from build123d import *
from build123d import SkipClean  # not in build123d's __all__

# Parameters (mm, degrees)
F1_DEPTH = 2
F2_R     = 6.75
F2_R_2   = 4
F3_DEPTH = 0.7
F4_SIZE2 = 1.5
F4_SIZE  = 3


with BuildPart() as f1:
    # F0 (on Top) → F1 (new body)
    with BuildSketch(Plane.XY):
        with BuildLine():
            ThreePointArc((0, 8.25), (-8.25, 0), (0, -8.25))
            Line((0, -8.25), (0, -14))
            ThreePointArc((0, -14), (4.5374051759, -13.2443178107), (8.5849765979, -11.05885061))
            ThreePointArc((8.5849765979, -11.05885061), (17.2671345057, -6.3709601788), (27, -4.75))
            ThreePointArc((27, -4.75), (36.7328654943, -6.3709601788), (45.4150234021, -11.05885061))
            ThreePointArc((45.4150234021, -11.05885061), (49.4625948241, -13.2443178107), (54, -14))
            Line((54, -14), (54, -8.25))
            ThreePointArc((54, -8.25), (62.25, 0), (54, 8.25))
            Line((54, 8.25), (0, 8.25))
        make_face()
        with BuildLine():
            ThreePointArc((0, -4), (-2.8284271247, 2.8284271247), (4, 0))
            ThreePointArc((4, 0), (2.8284271247, -2.8284271247), (0, -4))
        make_face(mode=Mode.SUBTRACT)
        with BuildLine():
            Line((38.1630301369, -4.75), (38.1409883593, -4.75))
            ThreePointArc((38.1409883593, -4.75), (38.0236172708, -4.7067170267), (37.9060780323, -4.6638927855))
            ThreePointArc((37.9060780323, -4.6638927855), (27.0000000348, -2.75), (16.0939220331, -4.6638927618))
            ThreePointArc((16.0939220331, -4.6638927618), (8.6383214319, -0.3472662226), (14.1786574679, 6.25))
            Line((14.1786574679, 6.25), (39.8213425321, 6.25))
            ThreePointArc((39.8213425321, 6.25), (43.7988181762, 4.6024756442), (45.4463425321, 0.625))
            ThreePointArc((45.4463425321, 0.625), (43.1614486514, -3.9009602419), (38.1630301369, -4.75))
        make_face(mode=Mode.SUBTRACT)
        with BuildLine():
            ThreePointArc((58, 0), (56.8284271247, -2.8284271247), (54, -4))
            ThreePointArc((54, -4), (51.1715728753, 2.8284271247), (58, 0))
        make_face(mode=Mode.SUBTRACT)
    extrude(amount=F1_DEPTH)

    # F2 (on face) → F3 (join)
    with BuildSketch(Plane.XY.offset(2)):
        Circle(F2_R)
        Circle(F2_R_2, mode=Mode.SUBTRACT)
        with Locations((54, 0)):
            Circle(F2_R)
        with Locations((54, 0)):
            Circle(F2_R_2, mode=Mode.SUBTRACT)
    with SkipClean():  # cleaning this boolean's faces spoils the solid; the shape is the same uncleaned
        extrude(amount=F3_DEPTH)

    # F4
    f4_edges = [f1.edges().sort_by_distance(p)[0] for p in [
        (0, -11.125, 2),
        (54, -11.125, 2),
    ]]
    f4_side = f1.faces().sort_by_distance((49.702195, -12.544944, 2))[0]
    chamfer(f4_edges, length=F4_SIZE, length2=F4_SIZE2, reference=f4_side)


solid = f1.part
Work out the finished part from the listing and answer in its coordinate system (mm). A direction names the side the tool comes from. Coordinates: 2 decimals unless noted, no trailing zeros. Order: outer loops, then holes, each group sorted by start corner. A loop starts at its lowest first (then second) coordinate and runs counter-clockwise, first axis right, second up. Notation, with made-up numbers: (75.25, 1) - (92.25, 1) arc R28 ccw to (92.25, 21) - close; hole circle Ø9 at (63.5, 41.5). An arc over 180 degrees is marked (long way). Put each result on its own line as item: value. Start each with the question number.
1) For a pull along X with two mould halves and no side action, classify faces 4 (the cylindrical face through (49.401, -13.223, 0.986)), 5 (the flat face through (3, -3, 2.7)), 6 (the cylindrical face through (8.664, -0.482, 0.986)) as released by +X, released by -X, zero draft, split by the parting line, or undercut.
2) For faces 1 (the cylindrical face through (4.476, -13.265, 0.986)), 2 (the flat face through (27, 6.25, 1)), 3 (the cylindrical face through (47.257, 0.297, 2.345)), determine the directions among +Z, -Z, +X, -X, +Y, -Y from which every point of the face is accessible in a straight line to the end or side of a thin tool.
3) Find section D-D (x = 29.5). Give the vertices of the cut face in (y, z), plus the area to 3 significant figures.
4) Find section A-A (x = 52.5). Give the vertices of the cut face in (y, z), plus the area to 3 significant figures.
5) Find section B-B (z = 1.1). Give the vertices of the cut face in (x, y) (3 decimals), plus the area to 3 significant figures.
6) Find section C-C (y = 5.5). Give the vertices of the cut face in (x, z), plus the area to 3 significant figures.
7) Find the intervals of material crossed by line 1 (Y direction, x = 0, z = 2.35); line 2 (Y direction, x = 27.5, z = 0.1); line 3 (Z direction, x = 10, y = -8), in increasing order. Write a range as from..to.
8) Flat-ended cylindrical pins translate along their axes: pin 1 (1.6 mm diameter, centred on x = 29, z = 1, fed in from -Y); pin 2 (12 mm diameter, centred on x = 36, y = -3, fed in from +Z); pin 3 (1 mm diameter, centred on x = 36, z = 1, fed in from -Y). Find the tip coordinate at first contact, or state that the pin passes through.
Results list:
1. face 4: undercut
1. face 5: zero draft
1. face 6: undercut
2. face 1: +Z, -Z, -Y
2. face 2: +Z, -Z
2. face 3: +Z
3. outline: (-4.85, 0) - (-2.85, 0) - (-2.85, 2) - (-4.85, 2) - close; (6.25, 0) - (8.25, 0) - (8.25, 2) - (6.25, 2) - close
3. area: 8.01 mm^2
4. outline: (-13.92, 0) - (-3.71, 0) - (-3.71, 2.7) - (-6.58, 2.7) - (-6.58, 2) - (-8.11, 2) - (-8.11, 1.25) - (-13.92, 1.25) - close; (3.71, 0) - (8.25, 0) - (8.25, 2) - (6.58, 2) - (6.58, 2.7) - (3.71, 2.7) - close
4. area: 29.2 mm^2
5. outline: (0, 8.25) arc R8.25 ccw (long way) to (1.2, -8.162) - (1.2, -13.948) arc R14 ccw to (8.585, -11.059) arc R30.03 cw to (45.415, -11.059) arc R14 ccw to (52.8, -13.948) - (52.8, -8.162) arc R8.25 ccw (long way) to (54, 8.25) - close; hole circle Ø8 at (0, 0); hole (14.179, 6.25) arc R5.625 ccw (long way) to (16.094, -4.664) arc R32.03 cw to (37.906, -4.664) arc R32.03 cw to (38.141, -4.75) - (38.163, -4.75) arc R5.625 ccw (long way) to (39.821, 6.25) - close; hole circle Ø8 at (54, 0)
5. area: 666 mm^2
6. outline: (-6.15, 0) - (11.37, 0) - (11.37, 2) - (3.91, 2) - (3.91, 2.7) - (-3.91, 2.7) - (-3.91, 2) - (-6.15, 2) - close; (42.63, 0) - (60.15, 0) - (60.15, 2) - (57.91, 2) - (57.91, 2.7) - (50.09, 2.7) - (50.09, 2) - (42.63, 2) - close
6. area: 81.0 mm^2
7. line 1: y = -6.75..-4, 4..6.75
7. line 2: y = -4.75..-2.75, 6.25..8.25
7. line 3: z = 0..2
8. pin 1: stops at y = -4.88
8. pin 2: stops at z = 2
8. pin 3: stops at y = -6.29
